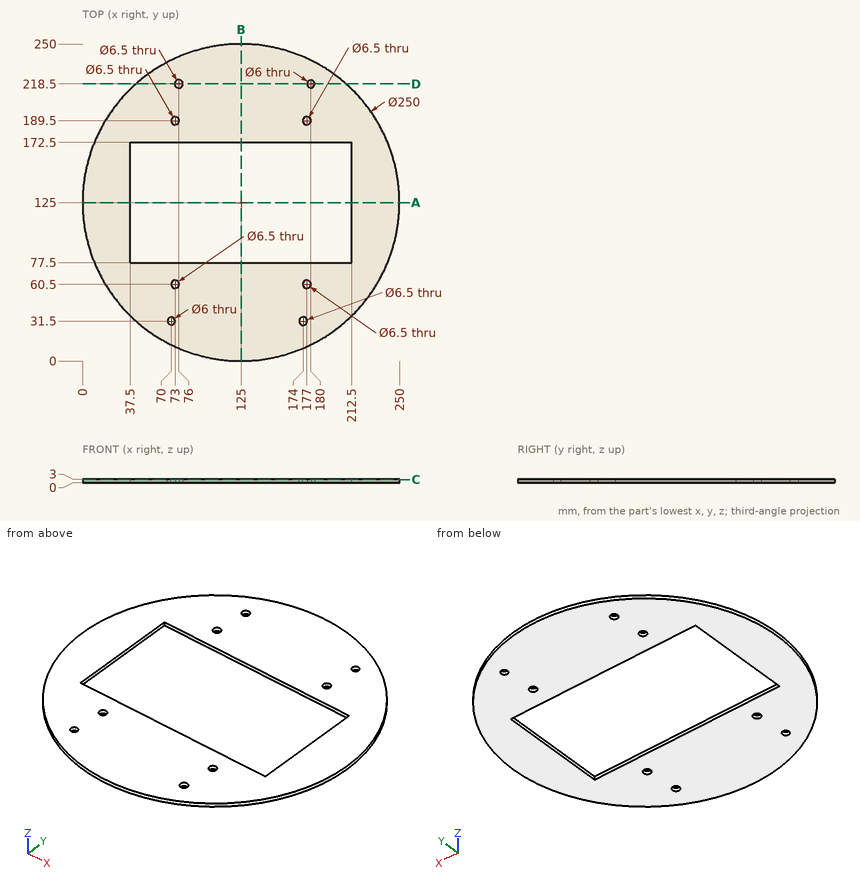
Print and shaded views of the part. All mm, measured from the part's lowest x, y and z. Give positions to 0.01 mm unless a question says otherwise; leave off trailing zeros. Write each loop counter-clockwise with the first axis right and the second up, starting at its lowest first coordinate (ties: lowest second). Pieces come first, ordered by that corner, then holes. Notation, with made-up numbers: (0, 56) - (47, 56) arc R23 cw to (47, 70) - close; hole circle Ø4 at (-4, -38.75). An arc over 180 degrees is marked (long way). One line per question, with ' | ' between items. Start each with the question number.
(1) Slice it at C-C on z = 2.45. Give the number of separate pieces and of enclosed holes in the cut face, plus the area to 3 significant figures.
(2) Pin check, flat tips, straight feed: P1, Ø8, axis at x = 180, y = 218.5, coming from the -Z side; P2, Ø4, axis at x = 177, y = 189.5, coming from the +Z side; P3, Ø1.5, axis at y = 49, z = 2, coming from the -X side; P4, Ø1.5, axis at y = 199, z = 2.5, coming from the -X side. Stop position of each tip, or through.
(3) Slice it at A-A on y = 125. Write the cut outline in (x, z), plus the area to 3 significant figures.
(4) Slice it at B-B on x = 125. Write the cut outline in (y, z), plus the area to 3 significant figures.
(5) Slice it at D-D on y = 218.5. Write the cut outline in (x, z).
(6) Wall check: line 1 along Y through (x, z) = (70, 1.3); line 2 along X through (y, z) = (189.5, 1.75); line 3 along X through (y, z) = (218.5, 1). Give the ranges that are in metal, low to high. Write a range as from..to.
Results below:
1) separate pieces: 1 | enclosed holes: 9 | area: 32,200 mm^2
2) P1: z = 0 | P2: through | P3: x = 25.19 | P4: x = 23.71
3) outline: (0, 0) - (37.5, 0) - (37.5, 3) - (0, 3) - close; (212.5, 0) - (250, 0) - (250, 3) - (212.5, 3) - close | area: 225 mm^2
4) outline: (0, 0) - (77.5, 0) - (77.5, 3) - (0, 3) - close; (172.5, 0) - (250, 0) - (250, 3) - (172.5, 3) - close | area: 465 mm^2
5) outline: (42.04, 0) - (72.75, 0) - (72.75, 3) - (42.04, 3) - close; (79.25, 0) - (177, 0) - (177, 3) - (79.25, 3) - close; (183, 0) - (207.96, 0) - (207.96, 3) - (183, 3) - close
6) line 1: 12.75..28.5, 34.5..59.25, 61.75..77.5, 172.5..188.25, 190.75..237.25 | line 2: 17.93..69.75, 76.25..173.75, 180.25..232.07 | line 3: 42.04..72.75, 79.25..177, 183..207.96
